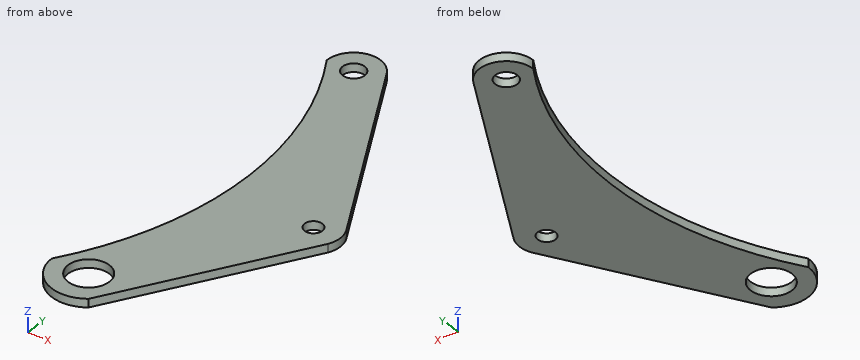
```python
from build123d import *

# Parameters (mm, degrees)
SKETCH1_R           = 7.8105
SKETCH1_R_2         = 3.3655
SKETCH1_R_3         = 4.191
BOSS_EXTRUDE1_DEPTH = 3.175


with BuildPart() as part:
    # Sketch1 → Boss-Extrude1 (new body)
    with BuildSketch(Plane.XY):
        with BuildLine():
            Line((8.98309661, 142.414532976), (49.565953559, 65.609056962))
            ThreePointArc((49.565953559, 65.609056962), (50.742856949, 60.862523985), (49.565953559, 56.115991009))
            Line((49.565953559, 56.115991009), (8.177790267, -11.326281223))
            ThreePointArc((8.177790267, -11.326281223), (-6.360706327, -12.437938536), (-13.97, 0))
            ThreePointArc((-13.97, 0), (7.886144716, 68.281846548), (-10.16, 137.668))
            ThreePointArc((-10.16, 137.668), (-2.445131739, 147.529385845), (8.98309661, 142.414532976))
        make_face()
        Circle(SKETCH1_R, mode=Mode.SUBTRACT)
        with Locations((40.582856949, 60.862523985)):
            Circle(SKETCH1_R_2, mode=Mode.SUBTRACT)
        with Locations((0, 137.668)):
            Circle(SKETCH1_R_3, mode=Mode.SUBTRACT)
    extrude(amount=BOSS_EXTRUDE1_DEPTH)


solid = part.part
```
Read the model definition and answer for the solid it produces. Units are mm, in the model's axes. Round coordinates to 2 decimals unless told otherwise and drop trailing zeros. Write each loop counter-clockwise with the first axis right and the second up, starting at its lowest first coordinate (ties: lowest second). Pieces come first, ordered by that corner, then holes. Notation, with made-up numbers: (62, -10) -> (115, -10) arc R19 ccw to (115, 21) -> close; hole circle Ø6 at (58.5, -29). An arc over 180 degrees is marked (long way). Answer in a Markdown table with one row per item. Add a question column.
1) Find section C-C, the plane z = 2.45. Determine the outline of the cut face in (x, y).
2) Consider line 1 (Y direction, x = -6, z = 0.3); line 2 (Y direction, x = -9, z = 2.3); line 3 (X direction, y = -6, z = 0.25). Determine where each line is inside the solid, lowest interval first.
3) Find section A-A, the plane x = 39. Determine the outline of the cut face in (y, z) (3 decimals), and give its area (3 significant figures).
4) Find section D-D, the plane y = 70.5. Determine the outline of the cut face in (x, z) (3 decimals).
5) Find section B-B, the plane x = 0. Determine the outline of the cut face in (y, z) (1 decimal), and give its area (3 significant figures).
6) Given P1, Ø6, axis at x = 12, y = 43, coming from the -Z side; P2, Ø1.5, axis at x = 35, z = 0.5, coming from the -Y side, each flat-ended and moving along its own axis, determine where each tip first touches the part or whether it passes through.
Findings below:
| question | item | result |
|---|---|---|
| 1 | outline | (-13.97, 0) arc R13.97 ccw to (8.18, -11.33) -> (49.57, 56.12) arc R10.16 ccw to (49.57, 65.61) -> (8.98, 142.41) arc R10.16 ccw to (-10.16, 137.67) arc R128.77 cw to start; hole circle Ø15.62 at (0, 0); hole circle Ø8.38 at (0, 137.67); hole circle Ø6.73 at (40.58, 60.86) |
| 2 | line 1 | -12.62 to -5, 5 to 13.58, 130.11 to 145.87 |
| 2 | line 2 | -10.68 to 8.01, 135.68 to 142.38 |
| 2 | line 3 | -12.62 to -5, 5 to 11.45 |
| 3 | outline | (38.899, 0) -> (57.892, 0) -> (57.892, 3.175) -> (38.899, 3.175) -> close; (63.833, 0) -> (85.606, 0) -> (85.606, 3.175) -> (63.833, 3.175) -> close |
| 3 | area | 129 mm² |
| 4 | outline | (7.928, 0) -> (46.982, 0) -> (46.982, 3.175) -> (7.928, 3.175) -> close |
| 5 | outline | (-14, 0) -> (-7.8, 0) -> (-7.8, 3.2) -> (-14, 3.2) -> close; (7.8, 0) -> (27.3, 0) -> (27.3, 3.2) -> (7.8, 3.2) -> close; (116.3, 0) -> (133.5, 0) -> (133.5, 3.2) -> (116.3, 3.2) -> close; (141.9, 0) -> (147.8, 0) -> (147.8, 3.2) -> (141.9, 3.2) -> close |
| 5 | area | 155 mm² |
| 6 | P1 | z = 0 |
| 6 | P2 | y = 31.16 |
